Verification items for the finished model (mm, model axes). A direction names the side the tool comes from. Give positions to 0.01 mm unless a question says otherwise; leave off trailing zeros. Order: outer loops, then holes, each group sorted by start corner. A loop starts at its lowest first (then second) coordinate and runs counter-clockwise, first axis right, second up. Notation, with made-up numbers: (82, 68.25) -> (123, 68.25) arc R16 cw to (123, 82.25) -> close; hole circle Ø3 at (21, 9). An arc over 180 degrees is marked (long way). Return JSON: item names as keys, results as strings. Group by question number.
(1) Depth check by flat-ended pin: pin 1 Ø3 at (x, z) = (77.8, -53.05) entering from -Y. Enter the tip coordinate at first touch or a pass-through.
(2) Release check for a two-part mould opening along X. For faces 3 (the face through (-1, 0, -1)), 4 (the face through (86.884, 0.74, -86.394)), 5 (the face through (76.61, 0.74, 76.87)), 6 (the face through (76.87, 0.74, -76.61)) record: pulls with the +X half, pulls with the -X half, needs draft (parallel to the pull), parting line crosses it, or undercut.
(3) Tool access check on faces 1 (the face through (81.98, 0.74, -62.89)), 2 (the face through (86.394, 0.74, 86.884)). Record the directions out of +Z, -Z, +X, -X, +Y, -Y that give a thin tool (end or side, any length) a straight path to the whole face; none if there is none.
(4) Thickness scan on line 1 along X through (y, z) = (0.5, -30); line 2 along X through (y, z) = (0.45, 80); line 3 along Z through (x, y) = (-72, 1.4). Record the ranges inside material, lowest first.
(5) Cross-section at B-B on y = 0.6. State how many separate pieces and enclosed holes the cut face has, then the cut area to 3 significant figures.
(6) Cross-section at A-A on z = -73.5. Enter the section's corners in (x, y), then the cut area to 3 significant figures.
from build123d import *

# Parameters (mm, degrees)
SKETCH2_R           = 1.6
SKETCH2_R_2         = 1.15
BOSS_EXTRUDE1_DEPTH = 1.5


with BuildPart() as part:
    # Sketch2 → Boss-Extrude1 (new body)
    with BuildSketch(Plane(origin=(0, 0, 0), x_dir=(1, 0, 0), z_dir=(0, 1, 0))):
        Polygon((104.138617256, -69.138617256), (104.138617256, 69.138617256), (69.138617256, 104.138617256), (-69.138617256, 104.138617256), (-104.138617256, 69.138617256), (-104.138617256, -69.138617256), (-69.138617256, -104.138617256), (69.138617256, -104.138617256), align=None)
        with Locations(Location((67.193180773, -91.941918115, 0), (0, 0, 270))):
            Circle(SKETCH2_R, mode=Mode.SUBTRACT)
        with Locations(Location((53.051045149, -77.799782491, 0), (0, 0, 270))):
            Circle(SKETCH2_R, mode=Mode.SUBTRACT)
        with Locations(Location((77.799782491, -53.051045149, 0), (0, 0, 270))):
            Circle(SKETCH2_R, mode=Mode.SUBTRACT)
        with Locations(Location((91.941918115, -67.193180773, 0), (0, 0, 270))):
            Circle(SKETCH2_R, mode=Mode.SUBTRACT)
        with Locations(Location((-67.193180773, -91.941918115, 0), (0, 0, 270))):
            Circle(SKETCH2_R, mode=Mode.SUBTRACT)
        with Locations(Location((-91.941918115, -67.193180773, 0), (0, 0, 270))):
            Circle(SKETCH2_R, mode=Mode.SUBTRACT)
        with Locations(Location((-77.799782491, -53.051045149, 0), (0, 0, 270))):
            Circle(SKETCH2_R, mode=Mode.SUBTRACT)
        with Locations(Location((-53.051045149, -77.799782491, 0), (0, 0, 270))):
            Circle(SKETCH2_R, mode=Mode.SUBTRACT)
        with Locations(Location((-77.799782491, 53.051045149, 0), (0, 0, 270))):
            Circle(SKETCH2_R, mode=Mode.SUBTRACT)
        with Locations(Location((-53.051045149, 77.799782491, 0), (0, 0, 270))):
            Circle(SKETCH2_R, mode=Mode.SUBTRACT)
        with Locations(Location((-67.193180773, 91.941918115, 0), (0, 0, 270))):
            Circle(SKETCH2_R, mode=Mode.SUBTRACT)
        with Locations(Location((-91.941918115, 67.193180773, 0), (0, 0, 270))):
            Circle(SKETCH2_R, mode=Mode.SUBTRACT)
        with Locations(Location((77.799782491, 53.051045149, 0), (0, 0, 270))):
            Circle(SKETCH2_R, mode=Mode.SUBTRACT)
        with Locations(Location((53.051045149, 77.799782491, 0), (0, 0, 270))):
            Circle(SKETCH2_R, mode=Mode.SUBTRACT)
        with Locations(Location((67.193180773, 91.941918115, 0), (0, 0, 270))):
            Circle(SKETCH2_R, mode=Mode.SUBTRACT)
        with Locations(Location((91.941918115, 67.193180773, 0), (0, 0, 270))):
            Circle(SKETCH2_R, mode=Mode.SUBTRACT)
        with Locations(Location((16, 30, 0), (0, 0, 270))):
            Circle(SKETCH2_R_2, mode=Mode.SUBTRACT)
        with Locations(Location((-16, 30, 0), (0, 0, 270))):
            Circle(SKETCH2_R_2, mode=Mode.SUBTRACT)
        with Locations(Location((-16, -30, 0), (0, 0, 270))):
            Circle(SKETCH2_R_2, mode=Mode.SUBTRACT)
        with Locations(Location((16, -30, 0), (0, 0, 270))):
            Circle(SKETCH2_R_2, mode=Mode.SUBTRACT)
        Polygon((86.285063865, -67.193180773), (77.799782491, -58.707899399), (58.707899399, -77.799782491), (67.193180773, -86.285063865), align=None, mode=Mode.SUBTRACT)
        Polygon((-67.193180773, -86.285063865), (-58.707899399, -77.799782491), (-77.799782491, -58.707899399), (-86.285063865, -67.193180773), align=None, mode=Mode.SUBTRACT)
        Polygon((-86.285063865, 67.193180773), (-77.799782491, 58.707899399), (-58.707899399, 77.799782491), (-67.193180773, 86.285063865), align=None, mode=Mode.SUBTRACT)
        Polygon((77.799782491, 58.707899399), (86.285063865, 67.193180773), (67.193180773, 86.285063865), (58.707899399, 77.799782491), align=None, mode=Mode.SUBTRACT)
    extrude(amount=BOSS_EXTRUDE1_DEPTH)


solid = part.part
Verdict:
{
 "1": {"pin 1": "through"},
 "2": {"face 3": "needs draft", "face 4": "pulls with the +X half", "face 5": "undercut", "face 6": "undercut"},
 "3": {"face 1": "+Y, -Y", "face 2": "+Z, +X, +Y, -Y"},
 "4": {"line 1": "-104.14 to -17.15, -14.85 to 14.85, 17.15 to 104.14", "line 2": "-93.28 to -73.48, -60.91 to 60.91, 73.48 to 93.28", "line 3": "-101.28 to -81.48, -64.51 to 64.51, 81.48 to 101.28"},
 "5": {"separate pieces": "1", "enclosed holes": "24", "area": "39,500 mm²"},
 "6": {"outline": "(-99.78, 0) -> (-79.98, 0) -> (-79.98, 1.5) -> (-99.78, 1.5) -> close; (-63.01, 0) -> (63.01, 0) -> (63.01, 1.5) -> (-63.01, 1.5) -> close; (79.98, 0) -> (99.78, 0) -> (99.78, 1.5) -> (79.98, 1.5) -> close", "area": "248 mm²"}
}
